Source: CAD feature listing. Evaluate the final solid. Frame: model axes, mm. A direction names the side the tool comes from. Round coordinates to 2 decimals unless told otherwise and drop trailing zeros. Return JSON: item names as keys, results as strings. Group by question number.
1) Contact query for flat-ended pins moving along their axis: P1, Ø8, axis at x = 5.08, y = 5.08, coming from the +Z side; P2, Ø1, axis at x = 11, z = 29.5, coming from the -Y side; P3, Ø6.5, axis at x = 5, y = 6.5, coming from the -Z side; P4, Ø2, axis at x = 0.5, z = 16.5, coming from the +Y side. Output: stop coordinate, or through.
2) Ray query, line 1 (X direction, y = 5.08, z = 24.5); line 2 (X direction, y = 11, z = -0.5); line 3 (Y direction, x = 5.08, z = 1.2). Return the intervals inside material, ascending. Write a range as from..to.
3) Access query for faces 4 (the cylindrical face through (8.88, 9.08, 9.39)), 5 (the cylindrical face through (-2.178, 12.318, 6.816)), 6 (the cylindrical face through (7.954, 6.272, 1.878)), 7 (the cylindrical face through (4, 8, 24)), 8 (the flat face through (3.78, 34.24, 55.43)). Directions: +Z, -Z, +X, -X, +Y, -Y. A direction counts if a zero-diameter tool reaches every point of the face in a straight line with its end or side. Return the directions, or none.
4) Mould query, pull axis Z, two halves, no side actions, for faces 1 (the cylindrical face through (4.67, 1.93, 12.61)), 2 (the flat face through (3.721, 36.82, 62.333)), 3 (the flat face through (-1, 12.7, 7)). Classes: pulls with the +Z half, pulls with the -Z half, needs draft (parallel to the pull), parting line crosses it, or undercut.
Autodesk Inventor part; units mm, degrees
ref_plane "YZ Plane" through (0, 0, 0) normal (1, 0, 0) x (0, 1, 0)
ref_plane "XZ Plane" through (0, 0, 0) normal (0, 1, 0) x (-1, 0, 0)
ref_plane "XY Plane" through (0, 0, 0) normal (0, 0, 1) x (1, 0, 0)
sketch "Sketch1" plane through (0, 0, 0) normal (0, 0, 1) x (1, 0, 0)
  line L0 (0, 0) -> (12.7, 0)
  line L1 (0, 0) -> (0, 12.7)
  arc A0 (12.7, 0) -> (0, 12.7) centre (0, 0) ccw
  circle A1 centre (5.08, 5.08) radius 3.1115
  dimension "d0" = 12.7
  dimension "d2" = 6.223
  dimension "d3" = 5.08
  dimension "d4" = 5.08
extrude "Extrusion1" add sketch "Sketch1" along normal blind 3.81
sketch "Sketch2" plane through (0, 0, 0) normal (0, 0, -1) x (-1, 0, 0)
  arc A0 (0, 12.7) -> (-12.7, 0) centre (0, 0) ccw
  line L0 (0, 12.7) -> (0, 0)
  line L1 (0, 12.7) -> (0, 0)
  line L2 (0, 0) -> (-12.7, 0)
  line L3 (-12.7, 0) -> (0, 0)
  line L4 (0, 12.7) -> (1.27, 12.7)
  line L5 (-12.7, 0) -> (-12.7, -1.27)
  line L6 (-11.43, -2.54) -> (1.27, -2.54)
  line L7 (2.54, -1.27) -> (2.54, 11.43)
  arc A1 (2.54, 11.43) -> (1.27, 12.7) centre (1.27, 11.43) ccw
  arc A2 (1.27, -2.54) -> (2.54, -1.27) centre (1.27, -1.27) ccw
  arc A3 (-12.7, -1.27) -> (-11.43, -2.54) centre (-11.43, -1.27) ccw
  point P0 (2.54, 12.7)
  point P1 (-12.7, -2.54)
  dimension "d7" = 2.54
  dimension "d8" = 2.54
  dimension "d9" = 1.27
extrude "Extrusion2" add sketch "Sketch2" along normal blind 5.08 and the other way blind 3.81 contours L4 A1 L7 A2 L6 A3 L5 L2 L0
sketch "Sketch3" plane through (0, 0, 3.81) normal (0, 0, 1) x (1, 0, 0)
  circle A0 centre (5.08, 5.08) radius 3.1115
  circle A1 centre (5.08, 5.08) radius 1.2
  arc A2 (12.7, 0) -> (0, 12.7) centre (0, 0) ccw
  arc A3 (12.7, 0) -> (0, 12.7) centre (0, 0) ccw
  line L0 (-1.27, -2.54) -> (11.43, -2.54)
  line L1 (12.7, -1.27) -> (12.7, 0)
  line L2 (-2.54, -1.27) -> (-2.54, 11.43)
  line L3 (-1.27, 12.7) -> (0, 12.7)
  arc A4 (11.43, -2.54) -> (12.7, -1.27) centre (11.43, -1.27) ccw
  arc A5 (-2.54, -1.27) -> (-1.27, -2.54) centre (-1.27, -1.27) ccw
  arc A6 (-1.27, 12.7) -> (-2.54, 11.43) centre (-1.27, 11.43) ccw
  point P0 (-2.54, -2.54)
  point P1 (12.7, -2.54)
  point P2 (-2.54, 12.7)
  dimension "d14" = 2.4
  dimension "d15" = 15.24
  dimension "d16" = 15.24
  dimension "d17" = 1.27
extrude "Extrusion3" add sketch "Sketch3" along normal blind 2.54 contours A0 | L1 A4 L0 A5 L2 A6 L3 A2
sketch "Sketch4" plane through (0, 0, 6.35) normal (0, 0, 1) x (1, 0, 0)
  line L0 (0, 0) -> (12.7, 0)
  line L1 (-1.27, 12.7) -> (0, 12.7)
  arc A0 (12.7, 0) -> (0, 12.7) centre (0, 0) ccw
  line L2 (0, 12.7) -> (-1.27, 12.7)
  line L3 (-2.54, 11.43) -> (-2.54, -1.27)
  line L4 (-1.27, -2.54) -> (11.43, -2.54)
  line L5 (12.7, -1.27) -> (12.7, 0)
  arc A1 (-1.27, 12.7) -> (-2.54, 11.43) centre (-1.27, 11.43) ccw
  arc A2 (-2.54, -1.27) -> (-1.27, -2.54) centre (-1.27, -1.27) ccw
  arc A3 (11.43, -2.54) -> (12.7, -1.27) centre (11.43, -1.27) ccw
  circle A4 centre (5.08, 5.08) radius 1.2
  circle A5 centre (5.08, 5.08) radius 3.175
  point P0 (-2.54, 12.7)
  point P1 (-2.54, -2.54)
  point P2 (12.7, -2.54)
  dimension "d20" = 15.24
  dimension "d21" = 15.24
  dimension "d22" = 1.27
  dimension "d23" = 6.35
extrude "Extrusion4" add sketch "Sketch4" along normal blind 12.7 contours L1 A0 L5 A3 L4 A2 L3 A1
sketch "Sketch5" plane through (-2.54, -1.27, -5.08) normal (-1, 0, 0) x (0, 0, 1)
  line L0 (24.13, 0) -> (0, 0)
  line L1 (24.13, 0) -> (69.0907, 35.9945)
  line L2 (24.13, 12.7) -> (0, 12.7)
  line L3 (24.13, 12.7) -> (62.8946, 43.7341)
  line L4 (69.0907, 35.9945) -> (62.8946, 43.7341)
  line L5 (24.13, 12.7) -> (24.13, 13.97)
  line L6 (24.13, 12.7) -> (24.13, 0)
  point P0 (5.08, 1.27)
  dimension "d26" = 141.32
  dimension "d27" = 141.32
  dimension "d28" = 57.594
extrude "Extrusion5" add sketch "Sketch5" against normal blind 12.7
sketch "Sketch6" plane through (0, 0, 19.05) normal (0, 0, 1) x (1, 0, 0)
  circle A0 centre (5.08, 5.08) radius 1.2
  circle A1 centre (5.08, 5.08) radius 3.1115
  point P0 (0, 0)
  dimension "d31" = 6.223
extrude "Extrusion6" cut sketch "Sketch6" along normal blind 12.7 contours A0 | A1
sketch "Sketch7" plane through (-2.54, 34.7245, 64.0107) normal (0, 0.6249702, 0.7806486) x (1, 0, 0)
  line L0 (8.0758, 9.9142) -> (12.7, 9.9142) construction
  line L1 (12.7, 0) -> (0, 0) construction
  line L2 (12.7, 9.9142) -> (0, 0) construction
  line L3 (0, 0) -> (0, 15.0805) construction
  line L4 (0, 9.9142) -> (12.7, 0) construction
  circle A0 centre (6.35, 4.9571) radius 2
  point P0 (2.54, 12.8971)
  dimension "d34" = 4
extrude "Extrusion7" cut sketch "Sketch7" against normal blind 7
fillet "Fillet1" radius 7.62 1 edges at (10.16, 26.947, 38.4323)
equation "\"d34\" = m3_heat_set_insert"
equation "\"d35\" = m3_heat_set_depth"
equation "\"m3_heat_set_insert\" = 4"
equation "\"m3_clearance\" = 3.4"
equation "\"m3_heat_set_depth\" = 7"
equation "\"robot_diameter\" = 354"
equation "\"hardboard_thickness\" = 5"
properties part number "display_top_support_left"
Geometry check:
{
 "1": {"P1": "z = 31.98", "P2": "through", "P3": "z = 0", "P4": "y = 12.7"},
 "2": {"line 1": "-2.54..1.97, 8.19..10.16", "line 2": "-2.54..0", "line 3": "-2.54..1.97, 8.19..11.64"},
 "3": {"face 4": "-Z, +X, +Y", "face 5": "-Z, -X, +Y", "face 6": "-Z", "face 7": "+Z", "face 8": "none"},
 "4": {"face 1": "undercut", "face 2": "pulls with the +Z half", "face 3": "needs draft"}
}
